Source: three-view drawing plus pictorial views. Frame: mm from the lowest corner of the part. A direction names the side the tool comes from. Give positions to 0.01 mm unless a question says otherwise; leave off trailing zeros. Order: outer loops, then holes, each group sorted by start corner. A loop starts at its lowest first (then second) coordinate and runs counter-clockwise, first axis right, second up.
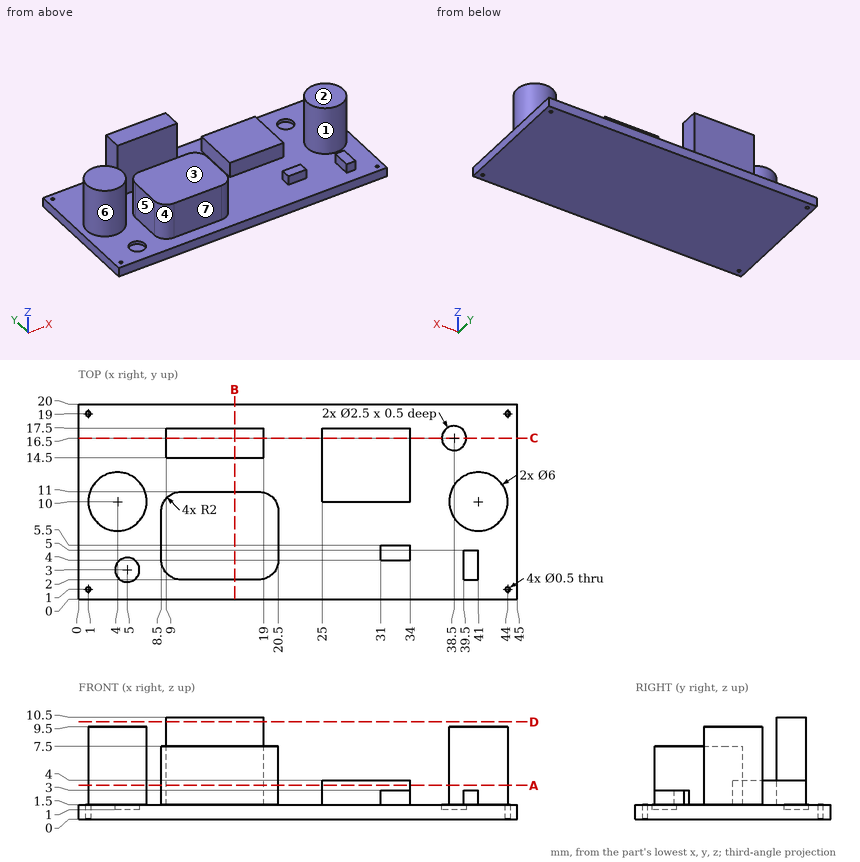
1) Section query A-A on z = 3.5. Output: boundary loops of the cut face in (x, y), and give its area (3 significant figures).
Checks:
outline: circle Ø6 at (4, 10); (8.5, 4) arc R2 ccw to (10.5, 2) - (18.5, 2) arc R2 ccw to (20.5, 4) - (20.5, 9) arc R2 ccw to (18.5, 11) - (10.5, 11) arc R2 ccw to (8.5, 9) - close; (9, 14.5) - (19, 14.5) - (19, 17.5) - (9, 17.5) - close; (25, 10) - (34, 10) - (34, 17.5) - (25, 17.5) - close; circle Ø6 at (41, 10)
area: 259 mm2
2) Reachability of the marked faces 5, 6 and 7 from +Z, -Z, +X, -X, +Y, -Y: full face, straight path, thin tool, end or side. Return the list, or none.
Checks:
face 5: +Z, +Y, -Y
face 6: +Z
face 7: +Z, +X, -X, -Y
3) First-contact query: pin 1 Ø5 at (x, z) = (15, 4.5) entering from +Y; pin 2 Ø3 at (y, z) = (11, 4.5) entering from +X; pin 3 Ø3 at (x, z) = (5, 3.5) entering from -Y. Flat tips, straight axial feed; report the tip coordinate or a pass-through.
Checks:
pin 1: stops at y = 17.5
pin 2: stops at x = 44
pin 3: stops at y = 7
4) Section query C-C on y = 16.5. Output: boundary loops of the cut face in (x, z), and give its area (3 significant figures).
Checks:
outline: (0, 0) - (45, 0) - (45, 1.5) - (39.75, 1.5) - (39.75, 1) - (37.25, 1) - (37.25, 1.5) - (34, 1.5) - (34, 4) - (25, 4) - (25, 1.5) - (19, 1.5) - (19, 10.5) - (9, 10.5) - (9, 1.5) - (0, 1.5) - close
area: 179 mm2
5) Ray query, L1, parallel to X at y = 19, z = 1.05; L2, parallel to Y at x = 1, z = 1.1; L3, parallel to X at y = 15, z = 3.5. Return the intervals inside material, ascending.
Checks:
L1: x = 0 to 0.75, 1.25 to 43.75, 44.25 to 45
L2: y = 0 to 0.75, 1.25 to 18.75, 19.25 to 20
L3: x = 9 to 19, 25 to 34
6) Section query B-B on x = 16. Output: boundary loops of the cut face in (y, z), and give its area (3 significant figures).
Checks:
outline: (0, 0) - (20, 0) - (20, 1.5) - (17.5, 1.5) - (17.5, 10.5) - (14.5, 10.5) - (14.5, 1.5) - (11, 1.5) - (11, 7.5) - (2, 7.5) - (2, 1.5) - (0, 1.5) - close
area: 111 mm2
7) Section query D-D on z = 10. Output: boundary loops of the cut face in (x, y), and give its area (3 significant figures).
Checks:
outline: (9, 14.5) - (19, 14.5) - (19, 17.5) - (9, 17.5) - close
area: 30.0 mm2
8) Pull-direction query (X, two-part tool) for the marked faces 1, 2, 3 and 4; classes: +X half, -X half, draft (parallel to the pull), parting line (faces both ways), or undercut.
Checks:
face 1: undercut
face 2: draft
face 3: undercut
face 4: -X half
